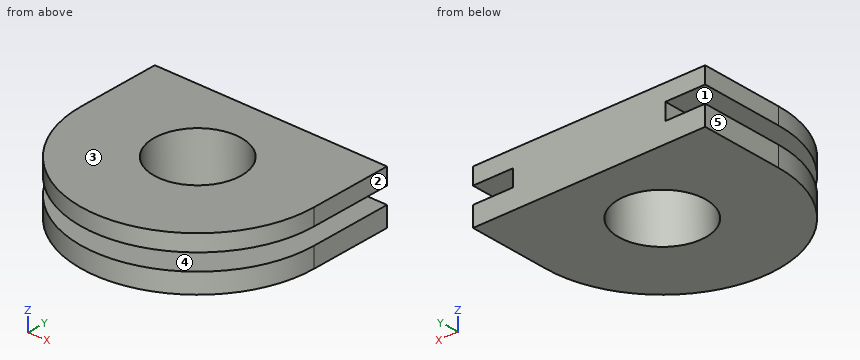
from build123d import *

# Parameters (mm, degrees)
PAD_DEPTH    = 3
PAD001_DEPTH = 2.5
PAD002_DEPTH = 2.5
SKETCH004_R  = 6.55
POCKET_DEPTH = 8.001


with BuildPart() as part:
    # Sketch001 → Pad (new body)
    with BuildSketch(Plane.XY):
        with BuildLine():
            Line((-17.5, 0), (17.5, 0))
            Line((17.5, 0), (17.5, -12.5))
            ThreePointArc((-17.5, -12.5), (0, -30), (17.5, -12.5))
            Line((-17.5, -12.5), (-17.5, 0))
        make_face()
    extrude(amount=PAD_DEPTH)

    # Sketch002 (on Face6 of Pad) → Pad001 (join)
    with BuildSketch(Plane.XY.offset(3)):
        with BuildLine():
            Line((11.5, 0), (11.5, -12.5))
            ThreePointArc((-11.5, -12.5), (0, -24), (11.5, -12.5))
            Line((-11.5, -12.5), (-11.5, 0))
            Line((-11.5, 0), (11.5, 0))
        make_face()
    extrude(amount=PAD001_DEPTH)

    # Sketch003 (on Face9 of Pad001) → Pad002 (join)
    with BuildSketch(Plane.XY.offset(5.5)):
        with BuildLine():
            Line((-17.5, 0), (17.5, 0))
            Line((17.5, 0), (17.5, -12.5))
            ThreePointArc((-17.5, -12.5), (0, -30), (17.5, -12.5))
            Line((-17.5, -12.5), (-17.5, 0))
        make_face()
    extrude(amount=PAD002_DEPTH)

    # Sketch004 (on Face12 of Pad002) → Pocket (cut, through all)
    with BuildSketch(Plane.XY.offset(8)):
        with Locations((0, -12.5)):
            Circle(SKETCH004_R)
    extrude(amount=-POCKET_DEPTH, mode=Mode.SUBTRACT)


solid = part.part
Here's how the part is built. I have some questions about the finished solid (model axes, mm). Face numbers are marked on the shaded views. A direction names the side the tool comes from. Coordinates: 2 decimals unless noted, no trailing zeros. Write each loop counter-clockwise with the first axis right and the second up, starting at its lowest first coordinate (ties: lowest second). Pieces come first, ordered by that corner, then holes.
1) If we section it at A-A (x = 0): List the corners of the cut face in (y, z) for me.
Filled in:
outline: (-30, 0) - (-19.05, 0) - (-19.05, 8) - (-30, 8) - (-30, 5.5) - (-24, 5.5) - (-24, 3) - (-30, 3) - close; (-5.95, 0) - (0, 0) - (0, 8) - (-5.95, 8) - close
2) I'm going to push a flat-ended pin straight in: pin 1 (2 mm diameter, centred on x = -2, z = 1, fed in from -Y). Where does the tip first touch, or does it pass through?
Filled in:
pin 1: stops at y = -29.97
3) If we section it at B-B (z = 5): List the corners of the cut face in (x, y) for me.
Filled in:
outline: (-11.5, -12.5) arc R11.5 ccw to (11.5, -12.5) - (11.5, 0) - (-11.5, 0) - close; hole circle Ø13.1 at (0, -12.5)
4) If we section it at D-D (y = -4): List the corners of the cut face in (x, z) for me, plus the area to 3 significant figures.
Filled in:
outline: (-17.5, 0) - (17.5, 0) - (17.5, 3) - (11.5, 3) - (11.5, 5.5) - (17.5, 5.5) - (17.5, 8) - (-17.5, 8) - (-17.5, 5.5) - (-11.5, 5.5) - (-11.5, 3) - (-17.5, 3) - close
area: 250 mm2
5) If we section it at C-C (y = -12): List the corners of the cut face in (x, z) for me.
Filled in:
outline: (-17.5, 0) - (-6.53, 0) - (-6.53, 8) - (-17.5, 8) - (-17.5, 5.5) - (-11.5, 5.5) - (-11.5, 3) - (-17.5, 3) - close; (6.53, 0) - (17.5, 0) - (17.5, 3) - (11.5, 3) - (11.5, 5.5) - (17.5, 5.5) - (17.5, 8) - (6.53, 8) - close
6) Which directions (+Z, -Z, +X, -X, +Y, -Y) give clear straight access to the entire face, cutting with the end or side of a thin tool? Please do the marked faces 4 and 5.
Filled in:
face 4: -Y
face 5: +Z, -Z, -X, +Y, -Y
7) Thinking about a two-plate mould opening in Z: for the marked faces 1, 2 and 3, which applies, +Z half, -Z half, draft (parallel to the pull), parting line (faces both ways), or undercut?
Filled in:
face 1: undercut
face 2: draft
face 3: +Z half
8) If I drill on line 1 (Y direction, x = 0, z = 3.25); line 2 (Z direction, x = -5, y = -23.5); line 3 (Y direction, x = 0, z = 6), over which ranges is the centre line in solid material (lowest first)?
Filled in:
line 1: y = -24 to -19.05, -5.95 to 0
line 2: z = 0 to 3, 5.5 to 8
line 3: y = -30 to -19.05, -5.95 to 0
